Design review of the part built by this model. Coordinates are the model's own, in mm. A direction names the side the tool comes from. Coordinates: 2 decimals unless noted, no trailing zeros. Use a Markdown table: item, result.
from build123d import *

# Parameters (mm, degrees)
SKETCH3_R          = 50
CUT_EXTRUDE1_DEPTH = 48
SKETCH4_R          = 43.75
CUT_EXTRUDE2_DEPTH = 52
CUT_EXTRUDE3_START = -10
SKETCH7_R          = 43.75
CUT_EXTRUDE3_DEPTH = 10
SKETCH8_R          = 11.625
SKETCH8_R_2        = 2.75
CUT_EXTRUDE4_DEPTH = 10


with BuildPart() as part:
    # Sketch2 → Revolve1 (revolve)
    with BuildSketch(Plane.XY, mode=Mode.PRIVATE) as revolve1_sk:
        Polygon((0, 0), (0, 63.5), (12.671353519, 50.828646481), (49.214586006, 50.828646481), (59.270211662, 44.337039427), (89.802920415, 44.337039427), (96.294527469, 50.828646481), (101.628646481, 50.828646481), (114.3, 63.5), (114.3, 0), align=None)
    revolve(revolve1_sk.sketch.rotate(Axis((0, 0, 0), (1, 0, 0)), 90), axis=Axis((0, 0, 0), (1, 0, 0)))

    # Sketch3 → Cut-Extrude1 (cut)
    with BuildSketch(Plane.ZY):
        Circle(SKETCH3_R)
    extrude(amount=-CUT_EXTRUDE1_DEPTH, mode=Mode.SUBTRACT)

    # Sketch4 → Cut-Extrude2 (cut)
    with BuildSketch(Plane(origin=(114.3, 0, 0), x_dir=(0, 0, -1), z_dir=(1, 0, 0))):
        Circle(SKETCH4_R)
    extrude(amount=-CUT_EXTRUDE2_DEPTH, mode=Mode.SUBTRACT)

    # Sketch5 → Cut-Revolve1 (revolve, cut)
    with BuildSketch(Plane.XY, mode=Mode.PRIVATE) as cut_revolve1_sk:
        Polygon((12.041253289, 50), (-0.277777226, 62.319030515), (-0.277777226, 50), align=None)
        Polygon((114.577777226, 62.319030515), (114.577777226, 50), (114.577777226, 45.7969371), (114.577777226, 42.174166746), (102.258746711, 42.174166746), (102.258746711, 45.7969371), (102.258746711, 50), align=None)
    revolve(cut_revolve1_sk.sketch.rotate(Axis((0, 0, 0), (1, 0, 0)), 90), axis=Axis((0, 0, 0), (1, 0, 0)), mode=Mode.SUBTRACT)

    # Sketch6 → Cut-Revolve2 (revolve, cut)
    with BuildSketch(Plane.XY, mode=Mode.PRIVATE) as cut_revolve2_sk:
        Polygon((55.706193059, 41.74129726), (47.124944427, 41.74129726), (47.124944427, 49.73979372), align=None)
    revolve(cut_revolve2_sk.sketch.rotate(Axis((0, 0, 0), (1, 0, 0)), 90), axis=Axis((0, 0, 0), (1, 0, 0)), mode=Mode.SUBTRACT)

    # Sketch7 → Cut-Extrude3 (cut)
    with BuildSketch(Plane.ZY.offset(-48).offset(CUT_EXTRUDE3_START)):
        with Locations(Location((0, 0, 0), (0, 0, 180))):
            Circle(SKETCH7_R)
    extrude(amount=CUT_EXTRUDE3_DEPTH, mode=Mode.SUBTRACT)

    # Sketch8 → Cut-Extrude4 (cut)
    with BuildSketch(Plane(origin=(62.3, 0, 0), x_dir=(0, 0, -1), z_dir=(1, 0, 0))):
        Circle(SKETCH8_R)
        with Locations((0, 30)):
            Circle(SKETCH8_R_2)
        with Locations((25.980762114, -15)):
            Circle(SKETCH8_R_2)
        with Locations((-25.980762114, -15)):
            Circle(SKETCH8_R_2)
    extrude(amount=-CUT_EXTRUDE4_DEPTH, mode=Mode.SUBTRACT)


solid = part.part
(1) Machinability: for faces 1 (the cylindrical face through (55.807, -29.568, 32.246)), 2 (the cylindrical face through (82.559, 29.568, 32.246)), 3 (the conical face through (12.056, 45.64, 23.738)), which of the approach directions +Z, -Z, +X, -X, +Y, -Y give a long, thin tool a straight path to every point of the face, cutting with its end or side? Answer none if there is none.
Determined:
| item | result |
|---|---|
| face 1 | -X |
| face 2 | +X |
| face 3 | none |
(2) Take a section at A-A on z = 0. State how many separate pieces and enclosed holes the cut face has, and give its area (3 significant figures).
Determined:
| item | result |
|---|---|
| separate pieces | 3 |
| enclosed holes | 0 |
| area | 619 mm2 |
(3) Draft analysis for pull direction X (two halves, no side actions). For faces 4 (the flat face through (102.259, 44, 0)), 5 (the cylindrical face through (98.999, 30.928, -40.336)), 6 (the cylindrical face through (60.18, 32.727, 0.358)), state which applies: +X half, -X half, draft (parallel to the pull), parting line (faces both ways), or undercut.
Determined:
| item | result |
|---|---|
| face 4 | +X half |
| face 5 | undercut |
| face 6 | draft |
(4) For L1, parallel to Y at x = 60.5, z = 0 (3 decimals); L2, parallel to Y at x = 31, z = 0; L3, parallel to X at y = 23.5, z = -57, list the stretches that pass through material, from the lowest coordinate up. Write a range as from..to.
Determined:
| item | result |
|---|---|
| L1 | -44.337..-11.625, 11.625..27.25, 32.75..44.337 |
| L2 | -50.83..-50, 50..50.83 |
| L3 | 0.39..1.85, 112.45..113.91 |
(5) For pin 1 (7 mm diameter, centred on y = -15, z = 25.98, fed in from +X); pin 2 (3 mm diameter, centred on x = 61, y = -38.5, fed in from +Z); pin 3 (3 mm diameter, centred on x = 18, z = 2.5, fed in from -Y); pin 4 (10 mm diameter, centred on y = 45.5, z = 41, fed in from -X), all flat-tipped, find the tip position at first contact; note any pin that passes through.
Determined:
| item | result |
|---|---|
| pin 1 | x = 62.3 |
| pin 2 | z = 24.43 |
| pin 3 | y = -50.82 |
| pin 4 | x = 0 |
